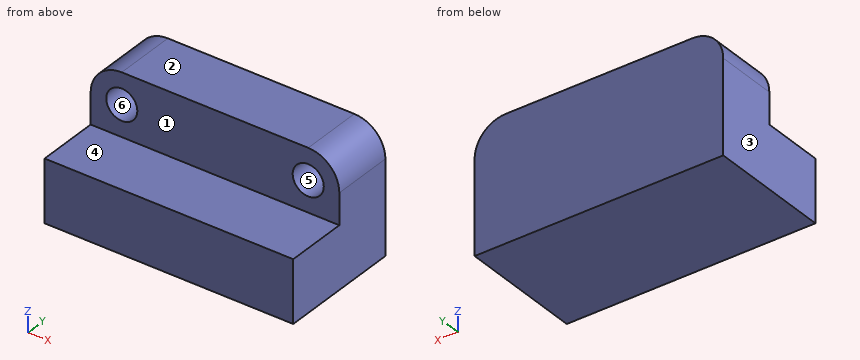
```python
from build123d import *

# Parameters (mm, degrees)
F1_DEPTH = 203.2
F2_W     = 76.2
F2_H     = 50.8
F3_DEPTH = 50.8
F4_R     = 25.4
F5_R     = 12.7
F6_DEPTH = 25.4


with BuildPart() as f1:
    # F0 (on Right) → F1 (new body)
    with BuildSketch(Plane.YZ):
        Polygon((14.799971, 3.178266), (-36.000029, 3.178266), (-36.000029, -47.621734), (65.599971, -47.621734), (65.599971, 3.178266), (65.599971, 53.978266), (14.799971, 53.978266), align=None)
    extrude(amount=F1_DEPTH)

    # F2 (on face) → F3 (cut)
    with BuildSketch(Plane(origin=(0, 0, -47.621734), x_dir=(1, 0, 0), z_dir=(0, 0, -1))):
        with Locations((38.1, 61.400029)):
            Rectangle(F2_W, F2_H)
        with Locations((241.3, 10.600029)):
            Rectangle(F2_W, F2_H)
    extrude(amount=-F3_DEPTH, mode=Mode.SUBTRACT)

    # F4
    f4_edges = [f1.edges().sort_by_distance(p)[0] for p in [
        (0, 40.199971, 53.978266),
        (203.2, 40.199971, 53.978266),
    ]]
    fillet(f4_edges, radius=F4_R)

    # F5 (on face) → F6 (cut)
    with BuildSketch(Plane.XZ.offset(-14.799971)):
        with Locations((25.4, 28.578266)):
            Circle(F5_R)
        with Locations((177.8, 28.578266)):
            Circle(F5_R)
    extrude(amount=-F6_DEPTH, mode=Mode.SUBTRACT)


solid = f1.part
```
Check sheet for the modelled part. Datum: model origin and axes. Units: mm. Face numbers are marked on the shaded views. A direction names the side the tool comes from. Give positions to 0.01 mm unless a question says otherwise; leave off trailing zeros. Loops run counter-clockwise (first coordinate to the right, second up) from the corner with the lowest first, then second, coordinate; pieces in that order, holes last. Notation, with made-up numbers: M 54,-11.75 L 79,-11.75 A27 ccw 79,15.25 Z; hole C 76,53 d8. An arc over 180 degrees is marked long. Answer in a Markdown table with one row per item.
1) Cross-section at D-D (y = 6). Enter the section's corners in (x, z), plus the area to 3 significant figures.
Solutions:
| item | result |
|---|---|
| outline | M 0,-47.62 L 203.2,-47.62 L 203.2,3.18 L 0,3.18 Z |
| area | 10,300 mm^2 |
2) Cross-section at C-C (z = 32). Enter the section's corners in (x, y), plus the area to 3 significant figures.
Solutions:
| item | result |
|---|---|
| outline | M 0.23,14.8 L 13.17,14.8 L 13.17,40.2 L 37.63,40.2 L 37.63,14.8 L 165.57,14.8 L 165.57,40.2 L 190.03,40.2 L 190.03,14.8 L 202.97,14.8 L 202.97,65.6 L 0.23,65.6 Z |
| area | 9,060 mm^2 |
3) Thickness scan on line 1 (Z direction, x = 177.8, y = 31); line 2 (X direction, y = 20, z = 38); line 3 (X direction, y = 34.5, z = 25). Record the ranges inside material, lowest first.
Solutions:
| item | result |
|---|---|
| line 1 | z = -47.62 to 15.88, 41.28 to 53.98 |
| line 2 | x = 1.81 to 16.88, 33.92 to 169.28, 186.32 to 201.39 |
| line 3 | x = 0 to 13.21, 37.59 to 165.61, 189.99 to 203.2 |
4) Depth check by flat-ended pin: pin 1 (20.5 mm diameter, centred on x = 183.5, z = 28.5, fed in from -Y); pin 2 (20.5 mm diameter, centred on x = 24.5, z = 29.5, fed in from -Y); pin 3 (10 mm diameter, centred on x = 34, z = 8, fed in from -Y). Enter the tip coordinate at first touch or a pass-through.
Solutions:
| item | result |
|---|---|
| pin 1 | stops at y = 14.8 |
| pin 2 | stops at y = 40.2 |
| pin 3 | stops at y = -36 |
5) Mould release check, pull along Z, two halves, no side actions. Record for the marked faces 3, 4, 5 and 6: released by +Z, released by -Z, zero draft, split by the parting line, or undercut.
Solutions:
| item | result |
|---|---|
| face 3 | zero draft |
| face 4 | released by +Z |
| face 5 | undercut |
| face 6 | undercut |
6) Tool access check on the marked faces 1 and 2. Record the directions out of +Z, -Z, +X, -X, +Y, -Y that give a thin tool (end or side, any length) a straight path to the whole face; none if there is none.
Solutions:
| item | result |
|---|---|
| face 1 | +Z, +X, -X, -Y |
| face 2 | +Z, +X, -X, +Y, -Y |
7) Cross-section at A-A (y = 28.5). Enter the section's corners in (x, z), plus the area to 3 significant figures.
Solutions:
| item | result |
|---|---|
| outline | M 0,-47.62 L 203.2,-47.62 L 203.2,28.58 A25.4 ccw 177.8,53.98 L 25.4,53.98 A25.4 ccw 0,28.58 Z; hole C 25.4,28.58 d25.4; hole C 177.8,28.58 d25.4 |
| area | 19,400 mm^2 |
8) Cross-section at B-B (x = 70). Enter the section's corners in (y, z), plus the area to 3 significant figures.
Solutions:
| item | result |
|---|---|
| outline | M -36,-47.62 L 65.6,-47.62 L 65.6,53.98 L 14.8,53.98 L 14.8,3.18 L -36,3.18 Z |
| area | 7,740 mm^2 |
